Check sheet for the modelled part. Datum: model origin and axes. Units: mm. Round coordinates to 2 decimals unless told otherwise and drop trailing zeros. Loops run counter-clockwise (first coordinate to the right, second up) from the corner with the lowest first, then second, coordinate; pieces in that order, holes last. Notation, with made-up numbers: (19.25, -21.5) - (78.25, -21.5) arc R13 cw to (78.25, -10.5) - close; hole circle Ø3 at (-29.5, 76.25). An arc over 180 degrees is marked (long way). Return JSON: item names as keys, results as strings.
from build123d import *

# Parameters (mm, degrees)
SALIENTE_EXTRUIR1_DEPTH = 3


with BuildPart() as part:
    # Croquis2 → Saliente-Extruir1 (new body)
    with BuildSketch(Plane(origin=(0, 0, 0), x_dir=(1, 0, 0), z_dir=(0, 1, 0))):
        with BuildLine():
            Line((-134.790190036, 51.201608082), (-137.430390036, 43.016906257))
            Line((-137.430390036, 43.016906257), (-134.575261492, 42.095906257))
            Line((-134.575261492, 42.095906257), (-131.935061492, 50.280608082))
            ThreePointArc((-131.935061492, 50.280608082), (-128.633444304, 46.478345774), (-128.480784458, 41.445))
            ThreePointArc((-128.480784458, 41.445), (-135, 0), (-128.480784458, -41.445))
            ThreePointArc((-128.480784458, -41.445), (-128.791366857, -46.852143005), (-132.662267215, -50.640254317))
            Line((-132.662267215, -50.640254317), (-135.302467215, -42.455552492))
            Line((-135.302467215, -42.455552492), (-138.157595759, -43.376552492))
            Line((-138.157595759, -43.376552492), (-135.618605817, -51.2475))
            ThreePointArc((-135.618605817, -51.2475), (-140.033424613, -49.810451014), (-142.756427176, -46.05))
            ThreePointArc((-142.756427176, -46.05), (-150, 0), (-142.756427176, 46.05))
            ThreePointArc((-142.756427176, 46.05), (-139.691309605, 50.045363436), (-134.790190036, 51.201608082))
        make_face()
    extrude(amount=SALIENTE_EXTRUIR1_DEPTH)


solid = part.part
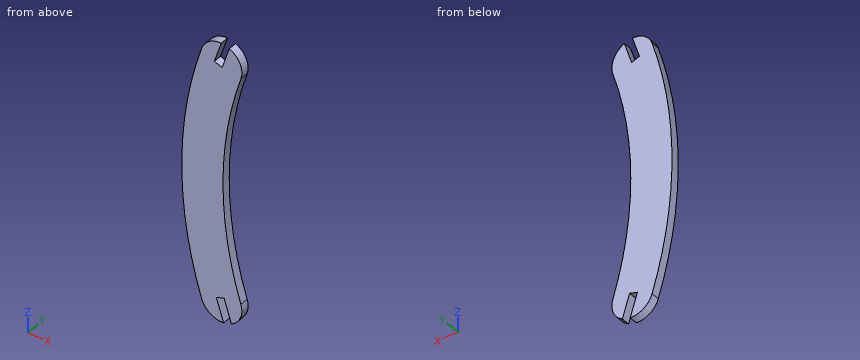
Q1. Depth check by flat-ended pin: P1, Ø1, axis at x = -131.5, y = 1, coming from the +Z side. Enter the tip coordinate at first touch or a pass-through.
Answer key:
{"P1": "stops at z = 50.32"}
Q2. Sectioned sample at B-B (z = 1.5). Enter the section's corners in (x, y).
Answer key:
{"outline": "(-149.99, 0) - (-134.99, 0) - (-134.99, 3) - (-149.99, 3) - close"}
Q3. Scan lines: probe 1 along X at (y, z) = (1.35, 0); probe 2 along X at (y, z) = (1.55, -46.5); probe 3 along X at (y, z) = (0.9, -12). Record each from-to range of solid material in increasing order. Write a range as [from, to].
Answer key:
{"probe 1": "x = [-150, -135]", "probe 2": "x = [-142.6, -136.31], [-133.15, -128.64]", "probe 3": "x = [-149.52, -134.47]"}
Q4. Sectioned sample at C-C (x = -140.5). Enter the section's corners in (y, z).
Answer key:
{"outline": "(0, -49.44) - (3, -49.44) - (3, 49.44) - (0, 49.44) - close"}
